For this review, take the finished solid that the model builds, in its own axes (mm). Coordinates: 2 decimals unless noted, no trailing zeros. Loops run counter-clockwise (first coordinate to the right, second up) from the corner with the lowest first, then second, coordinate; pieces in that order, holes last. Notation, with made-up numbers: M 75.25,29 L 91.25,29 A23 cw 91.25,52 Z; hole C 55.5,-5 d9. An arc over 180 degrees is marked long. Use one line per item in the form item = value.
```python
from build123d import *

# Parameters (mm, degrees)
SKETCH1_W           = 72
SKETCH1_H           = 72
SKETCH1_R           = 2.1
SKETCH1_R_2         = 7
BOSS_EXTRUDE1_DEPTH = 1.5875


with BuildPart() as part:
    # Sketch1 → Boss-Extrude1 (new, symmetric)
    with BuildSketch(Plane.XY):
        Rectangle(SKETCH1_W, SKETCH1_H)
        with Locations((-15.556349186, 15.556349186)):
            Circle(SKETCH1_R, mode=Mode.SUBTRACT)
        with Locations((15.556349186, 15.556349186)):
            Circle(SKETCH1_R, mode=Mode.SUBTRACT)
        with Locations((15.556349186, -15.556349186)):
            Circle(SKETCH1_R, mode=Mode.SUBTRACT)
        with Locations((-15.556349186, -15.556349186)):
            Circle(SKETCH1_R, mode=Mode.SUBTRACT)
        with Locations((26.162950904, 26.162950904)):
            Circle(SKETCH1_R, mode=Mode.SUBTRACT)
        with Locations((26.162950904, -26.162950904)):
            Circle(SKETCH1_R, mode=Mode.SUBTRACT)
        with Locations((-26.162950904, -26.162950904)):
            Circle(SKETCH1_R, mode=Mode.SUBTRACT)
        with Locations((-26.162950904, 26.162950904)):
            Circle(SKETCH1_R, mode=Mode.SUBTRACT)
        Circle(SKETCH1_R_2, mode=Mode.SUBTRACT)
    extrude(amount=BOSS_EXTRUDE1_DEPTH, both=True)


solid = part.part
```
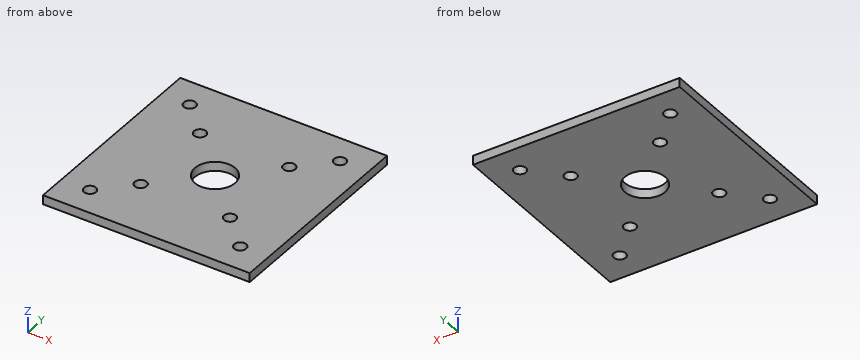
1. For pin 1 Ø3.5 at (x, y) = (-26.16, -26.16) entering from -Z, flat-tipped, find the tip position at first contact; note if it passes through.
Computed values:
pin_1 = through
2. Consider section A-A on x = 0. Write out the cut boundary in (y, z).
Computed values:
outline = M -36,-1.59 L -7,-1.59 L -7,1.59 L -36,1.59 Z; M 7,-1.59 L 36,-1.59 L 36,1.59 L 7,1.59 Z
3. Wall thickness on line 1 along X through (y, z) = (-26, 0.25); line 2 along X through (y, z) = (16, -0.3); line 3 along Y through (x, z) = (27.5, -1.1): over which ranges is each line inside the solid? List them lowest first. Write a range as from..to.
Computed values:
line_1 = -36..-28.26, -24.07..24.07, 28.26..36
line_2 = -36..-17.61, -13.5..13.5, 17.61..36
line_3 = -36..-27.78, -24.54..24.54, 27.78..36
4. Consider section C-C on z = -0.1. State how many separate pieces and enclosed holes the cut face has, plus the area to 3 significant figures.
Computed values:
separate_pieces = 1
enclosed_holes = 9
area = 4,920 mm2
